Could you check a few things on this model? Use its own coordinates, in mm. Round coordinates to 2 decimals unless told otherwise and drop trailing zeros. Order: outer loops, then holes, each group sorted by start corner. A loop starts at its lowest first (then second) coordinate and runs counter-clockwise, first axis right, second up. Notation, with made-up numbers: (-21.75, -12) -> (17.25, -12) arc R9 cw to (17.25, 0) -> close; hole circle Ø2 at (12.25, 77.5). An arc over 180 degrees is marked (long way). One line per question, with ' | ' between items.
```python
from build123d import *

# Parameters (mm, degrees)
SKETCH_1_R          = 1.5
EXTRUDE_1_DEPTH     = 3
SKETCH_3_R          = 1.5
CUT_EXTRUDE_1_DEPTH = 81.833161512
CUT_EXTRUDE_2_DEPTH = 81.833161512
FILLET_1_R          = 2


with BuildPart() as part:
    # 草图1 → 凸台-拉伸1 (new body)
    with BuildSketch(Plane(origin=(0, 0, 0), x_dir=(1, 0, 0), z_dir=(0, 1, 0))):
        Polygon((-65, 30), (65, 30), (65, -30), (-65, -30), (-75, -30), (-75, 30), align=None)
        with Locations(Location((-60, 10, 0), (0, 0, 270))):
            Circle(SKETCH_1_R, mode=Mode.SUBTRACT)
        with Locations(Location((-60, -10, 0), (0, 0, 270))):
            Circle(SKETCH_1_R, mode=Mode.SUBTRACT)
        with Locations(Location((-50, -24, 0), (0, 0, 270))):
            Circle(SKETCH_1_R, mode=Mode.SUBTRACT)
        with Locations(Location((-30, -24, 0), (0, 0, 270))):
            Circle(SKETCH_1_R, mode=Mode.SUBTRACT)
        with Locations(Location((-30, 24, 0), (0, 0, 90))):
            Circle(SKETCH_1_R, mode=Mode.SUBTRACT)
        with Locations(Location((-50, 24, 0), (0, 0, 90))):
            Circle(SKETCH_1_R, mode=Mode.SUBTRACT)
        with Locations(Location((-71, 21.5, 0), (0, 0, 270))):
            Circle(SKETCH_1_R, mode=Mode.SUBTRACT)
        with Locations(Location((-71, -21.5, 0), (0, 0, 270))):
            Circle(SKETCH_1_R, mode=Mode.SUBTRACT)
    extrude(amount=EXTRUDE_1_DEPTH)

    # 草图3 → 切除-拉伸1 (cut, through all)
    with BuildSketch(Plane.XZ):
        with Locations(Location((40, 4, 0), (0, 0, 270))):
            Circle(SKETCH_3_R)
        with Locations(Location((60, 4, 0), (0, 0, 270))):
            Circle(SKETCH_3_R)
        with Locations(Location((60, -4, 0), (0, 0, 90))):
            Circle(SKETCH_3_R)
        with Locations(Location((40, -4, 0), (0, 0, 90))):
            Circle(SKETCH_3_R)
    extrude(amount=-CUT_EXTRUDE_1_DEPTH, mode=Mode.SUBTRACT)

    # 草图4 → 切除-拉伸2 (cut, through all)
    with BuildSketch(Plane(origin=(0, 3, 0), x_dir=(1, 0, 0), z_dir=(0, 1, 0))):
        with BuildLine():
            Line((-10, 15), (-10, -15))
            ThreePointArc((-10, -15), (-15, -20), (-20, -15))
            Line((-20, -15), (-20, 15))
            ThreePointArc((-20, 15), (-15, 20), (-10, 15))
        make_face()
        with BuildLine():
            Line((10, 15), (10, -15))
            ThreePointArc((10, -15), (5, -20), (0, -15))
            Line((0, -15), (0, 15))
            ThreePointArc((0, 15), (5, 20), (10, 15))
        make_face()
        with BuildLine():
            Line((30, 15), (30, -15))
            ThreePointArc((30, -15), (25, -20), (20, -15))
            Line((20, -15), (20, 15))
            ThreePointArc((20, 15), (25, 20), (30, 15))
        make_face()
        with BuildLine():
            Line((47, 23), (53, 23))
            ThreePointArc((53, 23), (58, 18), (53, 13))
            Line((53, 13), (47, 13))
            ThreePointArc((47, 13), (42, 18), (47, 23))
        make_face()
        with BuildLine():
            Line((47, -23), (53, -23))
            ThreePointArc((53, -23), (58, -18), (53, -13))
            Line((53, -13), (47, -13))
            ThreePointArc((47, -13), (42, -18), (47, -23))
        make_face()
    extrude(amount=-CUT_EXTRUDE_2_DEPTH, mode=Mode.SUBTRACT)

    # 圆角1
    fillet_1_edges = [part.edges().sort_by_distance(p)[0] for p in [
        (65, 1.5, 30),
        (-75, 1.5, 30),
        (-75, 1.5, -30),
        (65, 1.5, -30),
    ]]
    fillet(fillet_1_edges, radius=FILLET_1_R)


solid = part.part
```
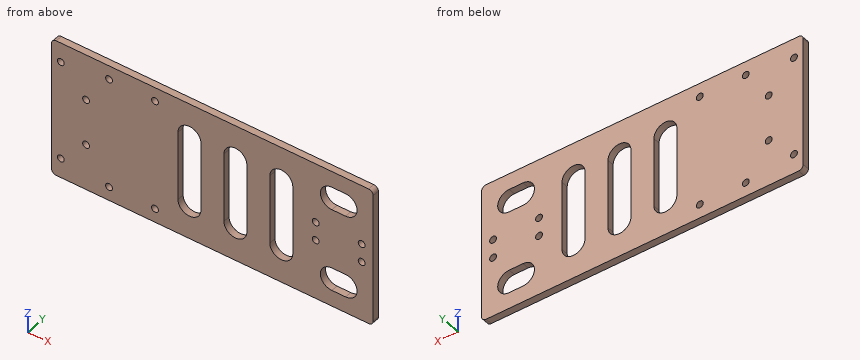
1. I want a section at B-B on x = 5. List the corners of the cut face in (y, z) for me.
From the geometry:
outline: (0, -30) -> (3, -30) -> (3, -20) -> (0, -20) -> close; (0, 20) -> (3, 20) -> (3, 30) -> (0, 30) -> close
2. I want a section at C-C on x = -30. List the corners of the cut face in (y, z) for me.
From the geometry:
outline: (0, -30) -> (3, -30) -> (3, -25.5) -> (0, -25.5) -> close; (0, -22.5) -> (3, -22.5) -> (3, 22.5) -> (0, 22.5) -> close; (0, 25.5) -> (3, 25.5) -> (3, 30) -> (0, 30) -> close
3. I want a section at A-A on z = 18. List the corners of the cut face in (x, y) for me.
From the geometry:
outline: (-75, 0) -> (-19, 0) -> (-19, 3) -> (-75, 3) -> close; (-11, 0) -> (1, 0) -> (1, 3) -> (-11, 3) -> close; (9, 0) -> (21, 0) -> (21, 3) -> (9, 3) -> close; (29, 0) -> (42, 0) -> (42, 3) -> (29, 3) -> close; (58, 0) -> (65, 0) -> (65, 3) -> (58, 3) -> close
4. I need wall thicknesses on probe 1 along X at (y, z) = (2.05, 12); probe 2 along X at (y, z) = (0.8, 10); probe 3 along X at (y, z) = (2, 4). Which ranges of each line are inside material? Lowest first, please.
From the geometry:
probe 1: x = -75 to -20, -10 to 0, 10 to 20, 30 to 65 | probe 2: x = -75 to -61.5, -58.5 to -20, -10 to 0, 10 to 20, 30 to 65 | probe 3: x = -75 to -20, -10 to 0, 10 to 20, 30 to 38.5, 41.5 to 58.5, 61.5 to 65
5. I want a section at D-D on z = 10. List the corners of the cut face in (x, y) for me.
From the geometry:
outline: (-75, 0) -> (-61.5, 0) -> (-61.5, 3) -> (-75, 3) -> close; (-58.5, 0) -> (-20, 0) -> (-20, 3) -> (-58.5, 3) -> close; (-10, 0) -> (0, 0) -> (0, 3) -> (-10, 3) -> close; (10, 0) -> (20, 0) -> (20, 3) -> (10, 3) -> close; (30, 0) -> (65, 0) -> (65, 3) -> (30, 3) -> close
